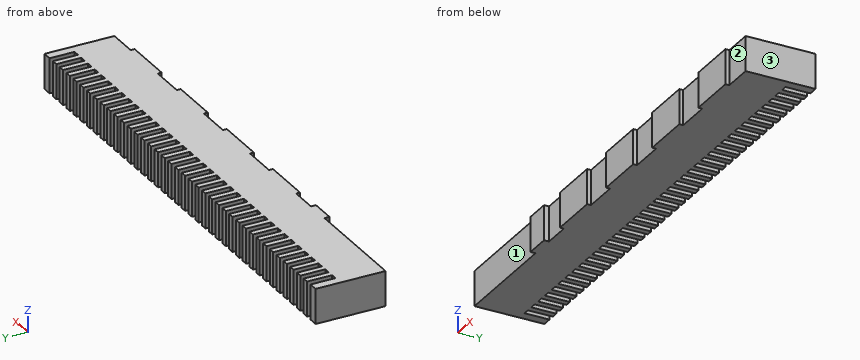
from build123d import *

# Parameters (mm, degrees)
SKETCH1_W           = 200
SKETCH1_H           = 14
BOSS_EXTRUDE1_DEPTH = 30
SKETCH2_W           = 12
SKETCH2_H           = 14
SKETCH2_W_2         = 14
SKETCH2_W_3         = 11
SKETCH2_W_4         = 45
CUT_EXTRUDE1_DEPTH  = 2
SKETCH3_W           = 20
SKETCH3_H           = 14
CUT_EXTRUDE2_DEPTH  = 0.435
CUT_EXTRUDE4_DEPTH  = 203.721483815


with BuildPart() as part:
    # Sketch1 → Boss-Extrude1 (new body)
    with BuildSketch(Plane(origin=(0, 0, 0), x_dir=(1, 0, 0), z_dir=(0, 1, 0))):
        with Locations((100, 7)):
            Rectangle(SKETCH1_W, SKETCH1_H)
    extrude(amount=BOSS_EXTRUDE1_DEPTH)

    # Sketch2 → Cut-Extrude1 (cut)
    with BuildSketch(Plane.XZ):
        with Locations((194, -7)):
            Rectangle(SKETCH2_W, SKETCH2_H)
        with Locations((161, -7)):
            Rectangle(SKETCH2_W_2, SKETCH2_H)
        with Locations((127, -7)):
            Rectangle(SKETCH2_W_2, SKETCH2_H)
        with Locations((93, -7)):
            Rectangle(SKETCH2_W_2, SKETCH2_H)
        with Locations((60.5, -7)):
            Rectangle(SKETCH2_W_3, SKETCH2_H)
        with Locations((22.5, -7)):
            Rectangle(SKETCH2_W_4, SKETCH2_H)
    extrude(amount=-CUT_EXTRUDE1_DEPTH, mode=Mode.SUBTRACT)

    # Sketch3 → Cut-Extrude2 (cut)
    with BuildSketch(Plane.XZ):
        with Locations((76, -7)):
            Rectangle(SKETCH3_W, SKETCH3_H)
        with Locations((110, -7)):
            Rectangle(SKETCH3_W, SKETCH3_H)
        with Locations((144, -7)):
            Rectangle(SKETCH3_W, SKETCH3_H)
        with Locations((178, -7)):
            Rectangle(SKETCH3_W, SKETCH3_H)
    extrude(amount=-CUT_EXTRUDE2_DEPTH, mode=Mode.SUBTRACT)

    # Sketch5 → Cut-Extrude4 (cut, through all)
    with BuildSketch(Plane.XY):
        Polygon((3.75, 30), (3.75, 20), (6.25, 20), (6.25, 30), (8.75, 30), (8.75, 20), (11.25, 20), (11.25, 30), (13.75, 30), (13.75, 20), (16.25, 20), (16.25, 30), (18.75, 30), (18.75, 20), (21.25, 20), (21.25, 30), (23.75, 30), (23.75, 20), (26.25, 20), (26.25, 30), (28.75, 30), (28.75, 20), (31.25, 20), (31.25, 30), (33.75, 30), (33.75, 20), (36.25, 20), (36.25, 30), (38.75, 30), (38.75, 20), (41.25, 20), (41.25, 30), (43.75, 30), (43.75, 20), (46.25, 20), (46.25, 30), (48.75, 30), (48.75, 20), (51.25, 20), (51.25, 30), (53.75, 30), (53.75, 20), (56.25, 20), (56.25, 30), (58.75, 30), (58.75, 20), (61.25, 20), (61.25, 30), (63.75, 30), (63.75, 20), (66.25, 20), (66.25, 30), (68.75, 30), (68.75, 20), (71.25, 20), (71.25, 30), (73.75, 30), (73.75, 20), (76.25, 20), (76.25, 30), (78.75, 30), (78.75, 20), (81.25, 20), (81.25, 30), (83.75, 30), (83.75, 20), (86.25, 20), (86.25, 30), (88.75, 30), (88.75, 20), (91.25, 20), (91.25, 30), (93.75, 30), (93.75, 20), (96.25, 20), (96.25, 30), (98.75, 30), (98.75, 20), (101.25, 20), (101.25, 30), (103.75, 30), (103.75, 20), (106.25, 20), (106.25, 30), (108.75, 30), (108.75, 20), (111.25, 20), (111.25, 30), (113.75, 30), (113.75, 20), (116.25, 20), (116.25, 30), (118.75, 30), (118.75, 20), (121.25, 20), (121.25, 30), (123.75, 30), (123.75, 20), (126.25, 20), (126.25, 30), (128.75, 30), (128.75, 20), (131.25, 20), (131.25, 30), (133.75, 30), (133.75, 20), (136.25, 20), (136.25, 30), (138.75, 30), (138.75, 20), (141.25, 20), (141.25, 30), (143.75, 30), (143.75, 20), (146.25, 20), (146.25, 30), (148.75, 30), (148.75, 20), (151.25, 20), (151.25, 30), (153.75, 30), (153.75, 20), (156.25, 20), (156.25, 30), (158.75, 30), (158.75, 20), (161.25, 20), (161.25, 30), (163.75, 30), (163.75, 20), (166.25, 20), (166.25, 30), (168.75, 30), (168.75, 20), (171.25, 20), (171.25, 30), (173.75, 30), (173.75, 20), (176.25, 20), (176.25, 30), (178.75, 30), (178.75, 20), (181.25, 20), (181.25, 30), (183.75, 30), (183.75, 20), (186.25, 20), (186.25, 30), (188.75, 30), (188.75, 20), (191.25, 20), (191.25, 30), (193.75, 30), (193.75, 20), (196.25, 20), (196.25, 30), (196.25, 37.451923055), (3.75, 37.451923055), align=None)
    extrude(amount=-CUT_EXTRUDE4_DEPTH, mode=Mode.SUBTRACT)


solid = part.part
Work out the finished part from the listing and answer in its coordinate system (mm). Face numbers are marked on the shaded views. A direction names the side the tool comes from. Give positions to 0.01 mm unless a question says otherwise; leave off trailing zeros. Use a Markdown table: item, result. Add a question column.
1. Flat-ended cylindrical pins translate along their axes: pin 1 Ø0.8 at (x, z) = (20, -5) entering from +Y; pin 2 Ø1.5 at (x, z) = (151, -9) entering from -Y (3 decimals); pin 3 Ø5.5 at (x, z) = (60, -5.5) entering from -Y. Find the tip coordinate at first contact, or state that the pin passes through.
2. For the marked faces 1, 2 and 3, determine the directions among +Z, -Z, +X, -X, +Y, -Y from which every point of the face is accessible in a straight line to the end or side of a thin tool.
3. Find the intervals of material crossed by probe 1 along Y at (x, z) = (182, -1.25) (3 decimals); probe 2 along Y at (x, z) = (85, -12) (3 decimals), in increasing order.
4. Section A-A on y = 22.5 is taken. State how many separate pieces and enclosed holes the cut face has, and give its area (4 significant figures).
Results below:
| question | item | result |
|---|---|---|
| 1 | pin 1 | stops at y = 20 |
| 1 | pin 2 | stops at y = 0.435 |
| 1 | pin 3 | stops at y = 2 |
| 2 | face 1 | +Z, -Z, -X, -Y |
| 2 | face 2 | +Z, -Z, +X, -Y |
| 2 | face 3 | +Z, -Z, +X, +Y, -Y |
| 3 | probe 1 | y = 0.435 to 30 |
| 3 | probe 2 | y = 0.435 to 20 |
| 4 | separate pieces | 40 |
| 4 | enclosed holes | 0 |
| 4 | area | 1,435 mm^2 |
